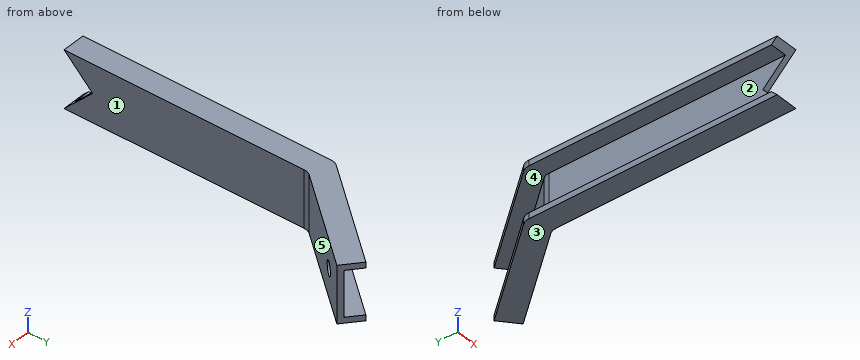
from build123d import *

# Parameters (mm, degrees)
BOSS_EXTRUDE1_DEPTH = 50
CUT_EXTRUDE1_REACH  = 338.776
SKETCH2_W           = 15
SKETCH2_H           = 40
CUT_EXTRUDE2_REACH  = 312.586
SKETCH3_W           = 15
SKETCH3_H           = 40
FILLET1_R           = 10
CUT_EXTRUDE3_REACH  = 210.165
CUT_EXTRUDE8_REACH  = 220.751
SKETCH7_R           = 6
CUT_EXTRUDE9_START  = -20
CUT_EXTRUDE9_DEPTH  = 20


with BuildPart() as part:
    # Sketch1 → Boss-Extrude1 (new body)
    with BuildSketch(Plane.XY):
        Polygon((10, -141.968058968), (10, 87.392238689), (78.367081497, 168.868953678), (63.046192634, 181.724705872), (-10, 94.671643375), (-10, -141.968058968), align=None)
    extrude(amount=BOSS_EXTRUDE1_DEPTH)

    # Cut-Extrude1: up to this plane
    cut_extrude1_end = Plane(origin=(-10, 94.671643375, 50), z_dir=(0.7660444431189772, -0.6427876096865403, 0))
    # Sketch2 → Cut-Extrude1 (cut, up to the surface)
    with BuildSketch(Plane.XZ.offset(141.968058968), mode=Mode.PRIVATE) as cut_extrude1_sk1:
        with Locations((-2.5, 25)):
            Rectangle(SKETCH2_W, SKETCH2_H)
    cut_extrude1_tool1 = split(extrude(cut_extrude1_sk1.sketch, amount=-CUT_EXTRUDE1_REACH, mode=Mode.PRIVATE), bisect_by=cut_extrude1_end, keep=Keep.BOTH, mode=Mode.PRIVATE)
    add(cut_extrude1_tool1.solids().sort_by_distance((-2.5, -141.968059, 25))[0], mode=Mode.SUBTRACT)

    # Cut-Extrude2: up to this plane
    cut_extrude2_end = Plane(origin=(5, 181.726705872, 45), z_dir=(-1, 0, 0))
    # Sketch3 → Cut-Extrude2 (cut, up to the surface)
    with BuildSketch(Plane(origin=(115.531117716, 137.684624594, 0), x_dir=(0.766044443118977, -0.6427876096865407, 0), z_dir=(0.6427876096865407, 0.766044443118977, 0)), mode=Mode.PRIVATE) as cut_extrude2_sk1:
        with Locations((-61.014203781, -25)):
            Rectangle(SKETCH3_W, SKETCH3_H)
    cut_extrude2_tool1 = split(extrude(cut_extrude2_sk1.sketch, amount=-CUT_EXTRUDE2_REACH, mode=Mode.PRIVATE), bisect_by=cut_extrude2_end, keep=Keep.BOTH, mode=Mode.PRIVATE)
    add(cut_extrude2_tool1.solids().sort_by_distance((68.791526, 176.903799, 25))[0], mode=Mode.SUBTRACT)

    # Fillet1
    fillet1_edges = [part.edges().sort_by_distance(p)[0] for p in [
        (-10, 94.671643375, 47.5),
        (10, 87.392238689, 25),
        (-10, 94.671643375, 2.5),
        (5, 89.212089861, 25),
    ]]
    fillet(fillet1_edges, radius=FILLET1_R)

    # Sketch4 → Cut-Extrude3 (cut, up to next)
    with BuildSketch(Plane.ZY.offset(10), mode=Mode.PRIVATE) as cut_extrude3_sk1:
        Polygon((0, -141.968058968), (25, -102.081750499), (50, -141.968058968), align=None)
    cut_extrude3_tool1 = extrude(cut_extrude3_sk1.sketch, amount=-CUT_EXTRUDE3_REACH, mode=Mode.PRIVATE) & part.part
    add(cut_extrude3_tool1.solids().sort_by_distance((-10, -128.672623, 25))[0], mode=Mode.SUBTRACT)

    # Sketch7 → Cut-Extrude8 (cut, up to next)
    with BuildSketch(Plane(origin=(-40.994258434, 34.398267133, 0), x_dir=(0, 0, 1), z_dir=(-0.766044443118977, 0.6427876096865406, 0)), mode=Mode.PRIVATE) as cut_extrude8_sk1:
        with Locations(Location((25, 149.734512574, 0), (0, 0, 270))):
            Circle(SKETCH7_R)
    cut_extrude8_tool1 = extrude(cut_extrude8_sk1.sketch, amount=-CUT_EXTRUDE8_REACH, mode=Mode.PRIVATE) & part.part
    add(cut_extrude8_tool1.solids().sort_by_distance((55.253231, 149.101558, 25))[0], mode=Mode.SUBTRACT)

    # Sketch10 → Cut-Extrude9 (cut)
    with BuildSketch(Plane.ZY.offset(10).offset(CUT_EXTRUDE9_START)):
        Polygon((50, -127.0817505), (25, -102.081750499), (0, -127.081750499), (0, -141.968058968), (50, -141.968058968), align=None)
    extrude(amount=CUT_EXTRUDE9_DEPTH, mode=Mode.SUBTRACT)


solid = part.part
Build history of the part. All positions in model axes, mm. Face numbers are marked on the shaded views. A direction names the side the tool comes from. Coordinates: 2 decimals unless noted, no trailing zeros. Order: outer loops, then holes, each group sorted by start corner. A loop starts at its lowest first (then second) coordinate and runs counter-clockwise, first axis right, second up. Notation, with made-up numbers: (22, 80) - (76, 80) arc R26 ccw to (76, 101) - close; hole circle Ø1 at (32, 69). An arc over 180 degrees is marked (long way). Put each result on its own line as item: value.
1. Saw through at A-A (y = 52.5). Write the cut outline in (x, z).
Answer sheet:
outline: (-10, 0) - (10, 0) - (10, 50) - (-10, 50) - (-10, 45) - (5, 45) - (5, 5) - (-10, 5) - close
2. Saw through at B-B (z = 13). Write the cut outline in (x, y).
Answer sheet:
outline: (5, -114.08) - (10, -114.08) - (10, 83.75) arc R10 cw to (12.34, 90.18) - (78.37, 168.87) - (74.54, 172.08) - (7.34, 92) arc R10 ccw to (5, 85.57) - close
3. Probe line 1 along Z through (x, y) = (-5, -46.5); line 2 along X through (y, z) = (82, 20.5); line 3 along X through (y, z) = (105, 25). List the from-to ranges inside material, lowest first. Write a range as [from, to].
Answer sheet:
line 1: z = [0, 5], [45, 50]
line 2: x = [5, 10]
line 3: x = [18.25, 24.77]
4. Drop flat-ended pins along their axis: P1, Ø10, axis at y = 118, z = 20.5, coming from the +X side; P2, Ø12, axis at y = -7.5, z = 25, coming from the -X side; P3, Ø2, axis at y = 131.5, z = 29.5, coming from the +X side. Give the stop position or say it passes through.
Answer sheet:
P1: stops at x = 39.88
P2: stops at x = 5
P3: stops at x = 47.85
5. Tool access for the marked faces 4 and 5: list every direction of +Z, -Z, +X, -X, +Y, -Y with a clear straight run to the whole face (end or side of a thin tool).
Answer sheet:
face 4: -X, +Y
face 5: +Z, -Z, +X, -Y
6. Pull direction Z, two halves, no side cores. Call the marked faces 1, 2 and 3: pulls with the +Z half, pulls with the -Z half, needs draft (parallel to the pull), parting line crosses it, or undercut.
Answer sheet:
face 1: needs draft
face 2: undercut
face 3: pulls with the -Z half
